For this review, use the dimensioned drawing (mm, ordinates from the lowest corner) and the shaded views. Round coordinates to 2 decimals unless told otherwise and drop trailing zeros. Write each loop counter-clockwise with the first axis right and the second up, starting at its lowest first coordinate (ties: lowest second). Pieces come first, ordered by that corner, then holes. Notation, with made-up numbers: (46.25, 48.25) -> (96.25, 48.25) arc R15 cw to (96.25, 52.25) -> close; hole circle Ø10 at (20, -27). An arc over 180 degrees is marked (long way). Write each question's results on one line, items separated by ' | '. Start each with the question number.
Item 1: Clearance check with a flat-ended pin moving along its axis: pin 1 (8 mm diameter, centred on x = 46.5, y = 17, fed in from -Z). State where the tip first meets the part, or that it passes through.
Item 2: Add section A-A (x = 38). State the section outline as (y, z) points, plus the area to 3 significant figures.
Item 3: Add section B-B (z = 37). State the section outline as (x, y) points (1 decimal).
Item 4: The part is to be moulded in two halves that separate along X. For the marked faces 1, 2, 3 and 4, say which applies: +X half, -X half, draft (parallel to the pull), parting line (faces both ways), or undercut.
Item 5: Add section C-C (x = 14.5). State the section outline as (y, z) points.
Item 6: To check wall thickness, follow line 1 along Y through (x, z) = (22, 54.5); line 2 along X through (y, z) = (5.5, 40) (1 decimal); line 3 along X through (y, z) = (19, 44.5) (1 decimal). State the ranges of each line that lie inside material, in increasing order.
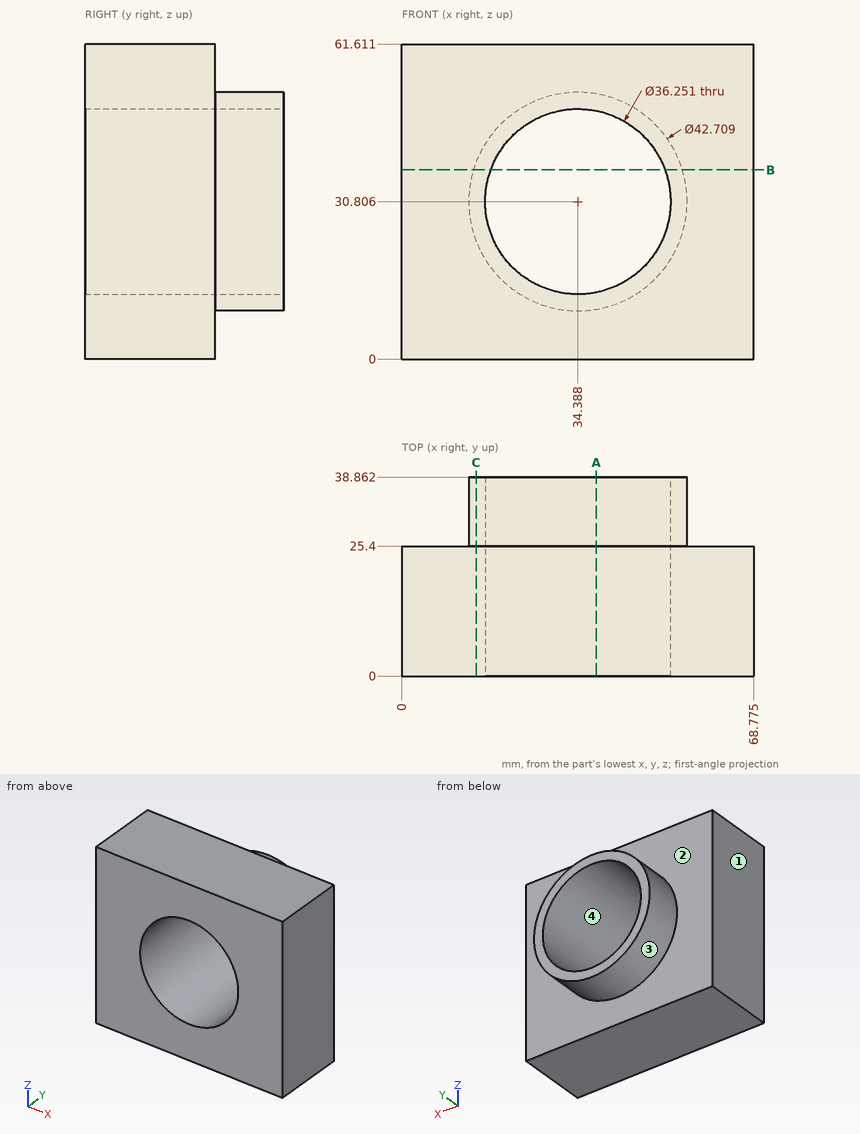
Responses:
1) pin 1: stops at z = 0
2) outline: (0, 0) -> (25.4, 0) -> (25.4, 9.76) -> (38.86, 9.76) -> (38.86, 13.04) -> (0, 13.04) -> close; (0, 48.57) -> (38.86, 48.57) -> (38.86, 51.85) -> (25.4, 51.85) -> (25.4, 61.61) -> (0, 61.61) -> close | area: 751 mm^2
3) outline: (0, 0) -> (17.4, 0) -> (17.4, 38.9) -> (14, 38.9) -> (14, 25.4) -> (0, 25.4) -> close; (51.4, 0) -> (68.8, 0) -> (68.8, 25.4) -> (54.8, 25.4) -> (54.8, 38.9) -> (51.4, 38.9) -> close
4) face 1: -X half | face 2: draft | face 3: parting line | face 4: undercut
5) outline: (0, 0) -> (25.4, 0) -> (25.4, 23.03) -> (38.86, 23.03) -> (38.86, 38.58) -> (25.4, 38.58) -> (25.4, 61.61) -> (0, 61.61) -> close
6) line 1: y = 0 to 25.4 | line 2: x = 0 to 18.8, 50 to 68.8 | line 3: x = 0 to 22.5, 46.3 to 68.8
